```python
from build123d import *

# Parameters (mm, degrees)
SKETCH1_W           = 12.5
SKETCH1_H           = 10.5
BOSS_EXTRUDE2_DEPTH = 15
BOSS_EXTRUDE3_DEPTH = 5


with BuildPart() as part:
    # Sketch1 → Boss-Extrude2 (new body)
    with BuildSketch(Plane(origin=(0, 0, 0), x_dir=(1, 0, 0), z_dir=(0, 1, 0))):
        Polygon((-36.75, -12.5), (-2, -12.5), (14.5, -12.5), (14.5, 2), (-2, 2), (-33.75, 2), (-33.75, 22), (-38.75, 22), (-38.75, -12.5), align=None)
        with Locations((6.25, -5.25)):
            Rectangle(SKETCH1_W, SKETCH1_H, mode=Mode.SUBTRACT)
    extrude(amount=BOSS_EXTRUDE2_DEPTH)

    # Sketch3 → Boss-Extrude3 (add)
    with BuildSketch(Plane(origin=(-33.75, 0, 0), x_dir=(0, 0, -1), z_dir=(1, 0, 0))):
        Polygon((2, 15), (2, 35), (-12.5, 35), (-12.5, -20), (2, -20), align=None)
    extrude(amount=-BOSS_EXTRUDE3_DEPTH)


solid = part.part
```
Can you work these out from the model? Positions are in its coordinate system, mm. A direction names the side the tool comes from. Coordinates: 2 decimals unless noted, no trailing zeros. Order: outer loops, then holes, each group sorted by start corner. A loop starts at its lowest first (then second) coordinate and runs counter-clockwise, first axis right, second up. Notation, with made-up numbers: (1, 81.25) - (38, 81.25) arc R28 ccw to (38, 117.25) - close; hole circle Ø1 at (-20, -22.75). An arc over 180 degrees is marked (long way). Answer in a Markdown table with one row per item.
1. For pin 1 (2.5 mm diameter, centred on x = -36, y = -14.5, fed in from -Z); pin 2 (12 mm diameter, centred on y = 6, z = -5, fed in from +X); pin 3 (16 mm diameter, centred on x = -12, z = 8, fed in from +Y); pin 4 (4.5 mm diameter, centred on y = -7.5, z = 3, fed in from +X), each with a flat end and sliding along its axis, tell me the tip position at first contact or that it passes through.
Reply:
| item | result |
|---|---|
| pin 1 | stops at z = -2 |
| pin 2 | stops at x = 14.5 |
| pin 3 | stops at y = 15 |
| pin 4 | stops at x = -33.75 |
2. If I drill on line 1 along Z through (x, y) = (7, 2); line 2 along X through (y, z) = (8, 8); line 3 along Y through (x, z) = (-5, 1.5), over which ranges is the centre line in solid material (lowest first)?
Reply:
| item | result |
|---|---|
| line 1 | z = -2 to 0, 10.5 to 12.5 |
| line 2 | x = -38.75 to 0, 12.5 to 14.5 |
| line 3 | y = 0 to 15 |
3. For faces 1 (the flat face through (-9, 7, -2)), 2 (the flat face through (-36, 25, -2)), 3 (the flat face through (0, 7, 5)), 4 (the flat face through (-33.75, -10, 5)), which set-ups out of +Z, -Z, +X, -X, +Y, -Y let a thin tool reach every point of the face, with its end or its side?
Reply:
| item | result |
|---|---|
| face 1 | -Z, +X, +Y, -Y |
| face 2 | -Z, +X, -X, +Y |
| face 3 | +Y, -Y |
| face 4 | +Z, -Z, +X, -Y |
4. Suppose I cut it at B-B (z = 4.5). Please give me the cut outline in (x, y).
Reply:
| item | result |
|---|---|
| outline | (-38.75, -20) - (-33.75, -20) - (-33.75, 0) - (0, 0) - (0, 15) - (-33.75, 15) - (-33.75, 35) - (-38.75, 35) - close; (12.5, 0) - (14.5, 0) - (14.5, 15) - (12.5, 15) - close |
5. Suppose I cut it at D-D (z = -5). Please give me the cut outline in (x, y).
Reply:
| item | result |
|---|---|
| outline | (-38.75, 0) - (-33.75, 0) - (-33.75, 15) - (-38.75, 15) - close |
6. Suppose I cut it at A-A (y = 10.5). Please give me the cut outline in (x, z).
Reply:
| item | result |
|---|---|
| outline | (-38.75, -22) - (-33.75, -22) - (-33.75, -2) - (14.5, -2) - (14.5, 12.5) - (-38.75, 12.5) - close; hole (0, 0) - (12.5, 0) - (12.5, 10.5) - (0, 10.5) - close |
7. If we mould it in two halves opening along Z, with no side actions, what happens to faces 5 (the flat face through (6, 7, 0)), 6 (the flat face through (-18, 8, 12.5)), 7 (the flat face through (-15, 0, 5))? For each: pulls with the +Z half, pulls with the -Z half, needs draft (parallel to the pull), parting line crosses it, or undercut.
Reply:
| item | result |
|---|---|
| face 5 | undercut |
| face 6 | pulls with the +Z half |
| face 7 | needs draft |
8. Suppose I cut it at C-C (x = -32.5). Please give me the cut outline in (y, z).
Reply:
| item | result |
|---|---|
| outline | (0, -2) - (15, -2) - (15, 12.5) - (0, 12.5) - close |
